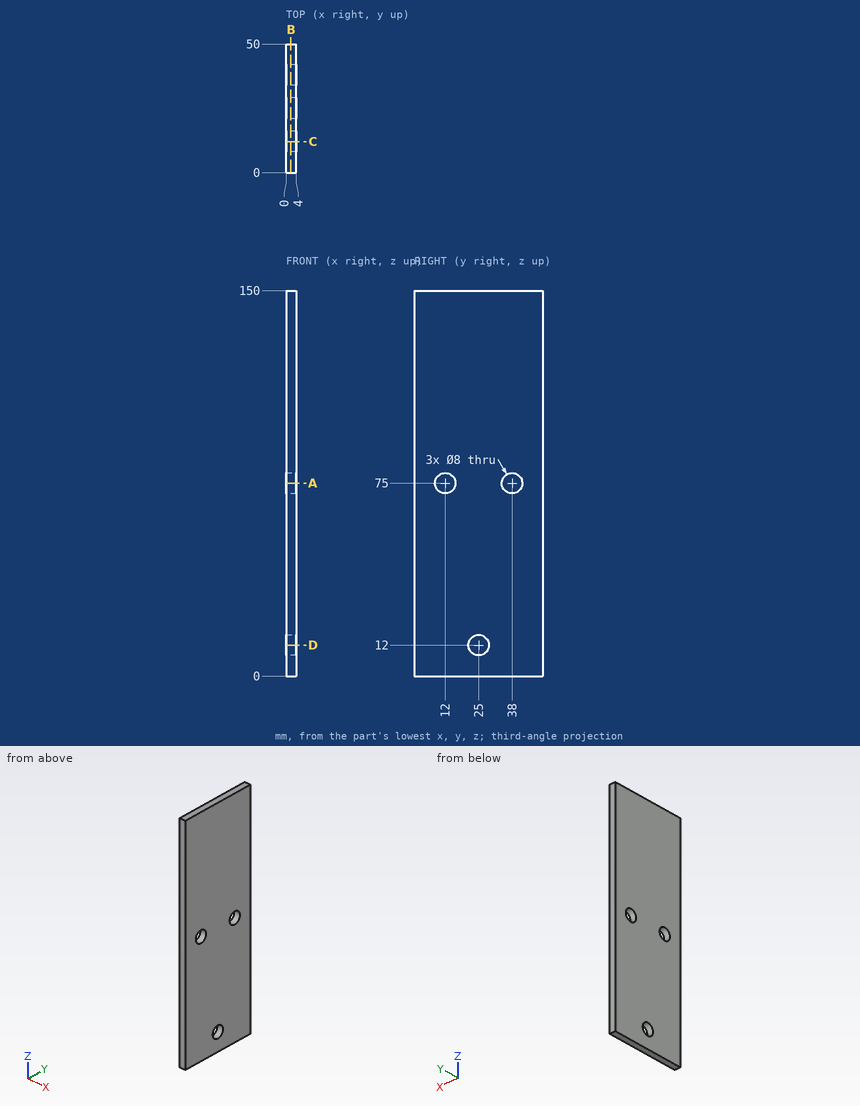
Part print with two shaded views. Sizes in mm from the minimum x, y, z corner. Give positions to 0.01 mm unless a question says otherwise; leave off trailing zeros. Order: outer loops, then holes, each group sorted by start corner. A loop starts at its lowest first (then second) coordinate and runs counter-clockwise, first axis right, second up.
(1) Saw through at D-D, the plane z = 12. Give the cut face in (x, y), then the cut area to 3 significant figures.
(2) Drill centre lines: L1, parallel to Y at x = 3, z = 75; L2, parallel to Y at x = 1.95, z = 12; L3, parallel to Y at x = 3.4, z = 8.5. Where is each one in solid material? Low to high.
(3) Saw through at C-C, the plane y = 12. Give the cut face in (x, z), then the cut area to 3 significant figures.
(4) Saw through at B-B, the plane x = 1.9. Give the cut face in (y, z), then the cut area to 3 significant figures.
(5) Saw through at A-A, the plane z = 75. Give the cut face in (x, y), then the cut area to 3 significant figures.
Results found:
1. outline: (0, 0) - (4, 0) - (4, 21) - (0, 21) - close; (0, 29) - (4, 29) - (4, 50) - (0, 50) - close
1. area: 168 mm2
2. L1: y = 0 to 8, 16 to 34, 42 to 50
2. L2: y = 0 to 21, 29 to 50
2. L3: y = 0 to 23.06, 26.94 to 50
3. outline: (0, 0) - (4, 0) - (4, 71) - (0, 71) - close; (0, 79) - (4, 79) - (4, 150) - (0, 150) - close
3. area: 568 mm2
4. outline: (0, 0) - (50, 0) - (50, 150) - (0, 150) - close; hole circle Ø8 at (12, 75); hole circle Ø8 at (25, 12); hole circle Ø8 at (38, 75)
4. area: 7,350 mm2
5. outline: (0, 0) - (4, 0) - (4, 8) - (0, 8) - close; (0, 16) - (4, 16) - (4, 34) - (0, 34) - close; (0, 42) - (4, 42) - (4, 50) - (0, 50) - close
5. area: 136 mm2
